from build123d import *

# Parameters (mm, degrees)
BOSS_EXTRUDE3_DEPTH     = 105
FILLET4_R               = 15
FILLET5_R               = 15
FILLET6_R               = 15
FILLET7_R               = 15
FILLET8_R               = 15
CUT_EXTRUDE3_DEPTH      = 1075.196909441
CUT_EXTRUDE3_DEPTH_BACK = 1075.196909441
SKETCH2_R               = 18.75


with BuildPart() as part:
    # Sketch1 → Boss-Extrude3 (new body)
    with BuildSketch(Plane.XY):
        Polygon((0, 93), (0, 78), (113.786796564, 78), (154.286796564, 37.5), (0, 37.5), (0, 0), (1065, 0), (1065, 37.5), (940.922649001, 37.5), (946.421161675, 48), (983.660254038, 112.5), (1065, 112.5), (1065, 127.5), (975, 127.5), (933.430780618, 55.5), (855, 55.5), (855, 37.5), (270, 37.5), (270, 55.5), (157.5, 55.5), (120, 93), align=None)
    extrude(amount=-BOSS_EXTRUDE3_DEPTH)

    # Fillet4
    fillet4_edges = [part.edges().sort_by_distance(p)[0] for p in [
        (157.5, 55.5, -52.5),
        (120, 93, -52.5),
        (940.922649001, 37.5, -52.5),
        (975, 127.5, -52.5),
    ]]
    fillet(fillet4_edges, radius=FILLET4_R)

    # Fillet5
    fillet5_edges = [part.edges().sort_by_distance(p)[0] for p in [
        (113.786796564, 78, -52.5),
    ]]
    fillet(fillet5_edges, radius=FILLET5_R)

    # Fillet6
    fillet6_edges = [part.edges().sort_by_distance(p)[0] for p in [
        (154.286796564, 37.5, -52.5),
    ]]
    fillet(fillet6_edges, radius=FILLET6_R)

    # Fillet7
    fillet7_edges = [part.edges().sort_by_distance(p)[0] for p in [
        (933.430780618, 55.5, -52.5),
    ]]
    fillet(fillet7_edges, radius=FILLET7_R)

    # Fillet8
    fillet8_edges = [part.edges().sort_by_distance(p)[0] for p in [
        (983.660254038, 112.5, -52.5),
    ]]
    fillet(fillet8_edges, radius=FILLET8_R)

    # Sketch2 → Cut-Extrude3 (cut, two sides: drawn at the far end of the back side and taken through both)
    with BuildSketch(Plane(origin=(0, 93, 0), x_dir=(1, 0, 0), z_dir=(0, 1, 0)).offset(-CUT_EXTRUDE3_DEPTH_BACK)):
        with Locations(Location((45, 52.5, 0), (0, 0, 270))):
            Circle(SKETCH2_R)
        with Locations(Location((1020, 52.5, 0), (0, 0, 270))):
            Circle(SKETCH2_R)
    extrude(amount=CUT_EXTRUDE3_DEPTH + CUT_EXTRUDE3_DEPTH_BACK, mode=Mode.SUBTRACT)


solid = part.part
Part model, mm, in its own coordinate system. A direction names the side the tool comes from. Coordinates: 2 decimals unless noted, no trailing zeros. Write each loop counter-clockwise with the first axis right and the second up, starting at its lowest first coordinate (ties: lowest second). Pieces come first, ordered by that corner, then holes. Notation, with made-up numbers: M -4.75,16.25 L 29.25,16.25 A15 ccw 29.25,31.25 Z; hole C 38,-1 d6. An arc over 180 degrees is marked long. Return JSON: item names as keys, results as strings.
1. Saw through at D-D, the plane x = 649. Write the cut outline in (y, z).
Determined:
{"outline": "M 0,-105 L 37.5,-105 L 37.5,0 L 0,0 Z"}
2. Flat gauge pins, fed straight in: pin 1 Ø10 at (y, z) = (54, -36.5) entering from +X; pin 2 Ø1 at (y, z) = (109, -69.5) entering from +X; pin 3 Ø4 at (y, z) = (72.5, -54.5) entering from +X. Where does each tip first touch, or does it go through?
Determined:
{"pin 1": "x = 952.82", "pin 2": "x = 983.32", "pin 3": "x = 961.72"}
3. 3-axis set-ups, long thin cutter, end or side, ignore diameter. For faces 4 (the face through (954.446, 91.899, -51.765)), 5 (the face through (65, 78, -52)), 6 (the face through (1005, 37.5, -40)), 7 (the face through (70, 93, -52)): which of +Z, -Z, +X, -X, +Y, -Y reach the whole face in a straight line?
Determined:
{"face 4": "+Z, -Z, +Y", "face 5": "+Z, -Z, -X", "face 6": "+Z, -Z, +X", "face 7": "+Z, -Z, -X, +Y"}
4. Saw through at B-B, the plane y = 17. Write the cut outline in (x, z).
Determined:
{"outline": "M 0,-105 L 1065,-105 L 1065,0 L 0,0 Z; hole C 45,-52.5 d37.5; hole C 1020,-52.5 d37.5"}
5. Saw through at A-A, the plane x = 1020. Write the cut outline in (y, z), then the cut area to 3 significant figures.
Determined:
{"outline": "M 0,-105 L 37.5,-105 L 37.5,-71.25 L 0,-71.25 Z; M 0,-33.75 L 37.5,-33.75 L 37.5,0 L 0,0 Z; M 112.5,-105 L 127.5,-105 L 127.5,-71.25 L 112.5,-71.25 Z; M 112.5,-33.75 L 127.5,-33.75 L 127.5,0 L 112.5,0 Z", "area": "3,540 mm²"}
6. Probe L1, parallel to X at y = 27, z = -52.5; L2, parallel to Z at x = 45, y = 24; L3, parallel to X at y = 82.75, z = -52.5. List the from-to ranges inside material, lowest first.
Determined:
{"L1": "0 to 26.25, 63.75 to 1001.25, 1038.75 to 1065", "L2": "-105 to -71.25, -33.75 to 0", "L3": "0 to 26.25, 63.75 to 130.25, 949.16 to 966.48"}
7. Pull direction Z, two halves, no side cores. Call faces 1 (the face through (525, 36, -105)), 2 (the face through (218, 55.5, -52)), 3 (the face through (60.81, 85.39, -42.42)): pulls with the +Z half, pulls with the -Z half, needs draft (parallel to the pull), parting line crosses it, or undercut.
Determined:
{"face 1": "pulls with the -Z half", "face 2": "needs draft", "face 3": "undercut"}
8. Saw through at C-C, the plane z = -52.5. Count the separate pieces of the cut face and the enclosed holes in it, then the cut area to 3 significant figures.
Determined:
{"separate pieces": "5", "enclosed holes": "0", "area": "45,100 mm²"}
